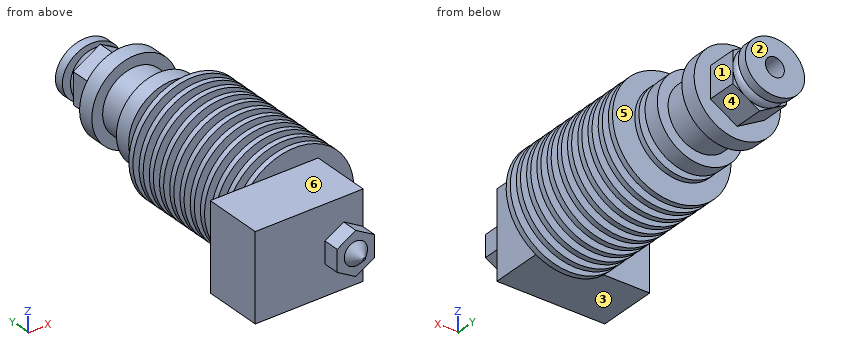
from build123d import *

# Parameters (mm, degrees)
SALIENTE_EXTRUIR1_DEPTH = 5.5
CROQUIS3_R              = 5
SALIENTE_EXTRUIR2_DEPTH = 2
REDONDEO1_R             = 2
CROQUIS4_RX             = 5.5
CROQUIS4_RY             = 5
SALIENTE_EXTRUIR3_DEPTH = 1.7
CROQUIS5_W              = 20
CROQUIS5_H              = 16
SALIENTE_EXTRUIR4_DEPTH = 11
SALIENTE_EXTRUIR5_START = 0.5
CROQUIS6_R              = 2.5
SALIENTE_EXTRUIR5_DEPTH = 0.5
SALIENTE_EXTRUIR6_DEPTH = 3
CROQUIS8_R              = 2.15
SALIENTE_EXTRUIR7_DEPTH = 2
SALIENTE_EXTRUIR7_TAPER = 44
CROQUIS9_R              = 1.75
CORTAR_EXTRUIR1_DEPTH   = 60


with BuildPart() as part:
    # Croquis1 → Revolución1 (revolve)
    with BuildSketch(Plane.XY, mode=Mode.PRIVATE) as revoluci_n1_sk:
        Polygon((0, 0), (0, 42), (8, 42), (8, 39), (6, 39), (6, 33), (8, 33), (8, 30), (4.5, 30), (4.5, 28.5), (8, 28.5), (8, 27.5), (4.5, 27.5), (4.5, 26), (11, 26), (11, 25), (4.5, 25), (4.5, 23.5), (11, 23.5), (11, 22.5), (4.5, 22.5), (4.541860465, 21), (11, 21), (11, 20), (4.569767442, 20), (4.611627907, 18.5), (11, 18.5), (11, 17.5), (4.639534884, 17.5), (4.681395349, 16), (11, 16), (11, 15), (4.709302326, 15), (4.751162791, 13.5), (11, 13.5), (11, 12.5), (4.779069767, 12.5), (4.820930233, 11), (11, 11), (11, 10), (4.848837209, 10), (4.890697674, 8.5), (11, 8.5), (11, 7.5), (4.918604651, 7.5), (4.960465116, 6), (11, 6), (11, 5), (4.988372093, 5), (5.030232558, 3.5), (11, 3.5), (11, 2.5), (5.058139535, 2.5), (5.1, 1), (11, 1), (11, 0), (2.5, 0), (2.5, -0.5), (0, -0.5), align=None)
    revolve(revoluci_n1_sk.sketch.rotate(Axis((0, 0, 0), (0, 1, 0)), 90), axis=Axis((0, 0, 0), (0, 1, 0)))

    # Croquis2 → Saliente-Extruir1 (add)
    with BuildSketch(Plane(origin=(0, 42, 0), x_dir=(1, 0, 0), z_dir=(0, 1, 0))):
        Polygon((0, 5.773502692), (-5, 2.886751346), (-5, -2.886751346), (0, -5.773502692), (5, -2.886751346), (5, 2.886751346), align=None)
    extrude(amount=SALIENTE_EXTRUIR1_DEPTH)

    # Croquis3 → Saliente-Extruir2 (add)
    with BuildSketch(Plane(origin=(0, 47.5, 0), x_dir=(1, 0, 0), z_dir=(0, 1, 0))):
        with Locations(Location((0, 0, 0), (0, 0, 60))):
            Circle(CROQUIS3_R)
    extrude(amount=SALIENTE_EXTRUIR2_DEPTH)

    # Redondeo1
    redondeo1_edges = [part.edges().sort_by_distance(p)[0] for p in [
        (-2.5, 49.5, 4.330127019),
    ]]
    fillet(redondeo1_edges, radius=REDONDEO1_R - 0.0001)  # a hair under: the kernel refuses the full size

    # Croquis4 → Saliente-Extruir3 (add)
    with BuildSketch(Plane(origin=(0, 49.5, 0), x_dir=(1, 0, 0), z_dir=(0, 1, 0))):
        with Locations(Location((0, 0), (0, 0, -180))):
            Ellipse(CROQUIS4_RX, CROQUIS4_RY)
    extrude(amount=SALIENTE_EXTRUIR3_DEPTH)

    # Croquis5 → Saliente-Extruir4 (add)
    with BuildSketch(Plane(origin=(0, -0.5, 0), x_dir=(-1, 0, 0), z_dir=(0, -1, 0))):
        with Locations((6, 0)):
            Rectangle(CROQUIS5_W, CROQUIS5_H)
    extrude(amount=SALIENTE_EXTRUIR4_DEPTH)

    # Croquis6 → Saliente-Extruir5 (add)
    with BuildSketch(Plane.XZ.offset(11.5).offset(SALIENTE_EXTRUIR5_START)):
        with Locations(Location((0, 0, 0), (0, 0, 270))):
            Circle(CROQUIS6_R)
    extrude(amount=-SALIENTE_EXTRUIR5_DEPTH)

    # Croquis7 → Saliente-Extruir6 (add)
    with BuildSketch(Plane.XZ.offset(12)):
        Polygon((0, -4), (3.464101615, -2), (3.464101615, 2), (0, 4), (-3.464101615, 2), (-3.464101615, -2), align=None)
    extrude(amount=SALIENTE_EXTRUIR6_DEPTH)

    # Croquis8 → Saliente-Extruir7 (add)
    with BuildSketch(Plane.XZ.offset(15)):
        Circle(CROQUIS8_R)
    extrude(amount=SALIENTE_EXTRUIR7_DEPTH, taper=SALIENTE_EXTRUIR7_TAPER)

    # Croquis9 → Cortar-Extruir1 (cut)
    with BuildSketch(Plane(origin=(0, 51.2, 0), x_dir=(1, 0, 0), z_dir=(0, 1, 0))):
        with Locations(Location((0, 0, 0), (0, 0, 270))):
            Circle(CROQUIS9_R)
    extrude(amount=-CORTAR_EXTRUIR1_DEPTH, mode=Mode.SUBTRACT)


solid = part.part
CAD build for the part. Positions are in the model's coordinates, mm. Face numbers are marked on the shaded views. A direction names the side the tool comes from. Coordinates: 2 decimals unless noted, no trailing zeros. Write each loop counter-clockwise with the first axis right and the second up, starting at its lowest first coordinate (ties: lowest second). Pieces come first, ordered by that corner, then holes. Notation, with made-up numbers: M 6,-17 L 54,-17 A22 cw 54,-8 Z; hole C 33.5,-21 d4. An arc over 180 degrees is marked long. Return JSON: item names as keys, results as strings.
Item 1: Which spindle directions (+Z, -Z, +X, -X, +Y, -Y) get a long thin tool onto all of the face, cutting with end or side? Do the marked faces 4, 5 and 6. Say none if no direction does.
Findings below:
{"face 4": "-Z, +X", "face 5": "none", "face 6": "+Z, +X, -X, -Y"}
Item 2: Slice it at B-B, the plane x = -14. Write the cut outline in (y, z), and give its area (3 significant figures).
Findings below:
{"outline": "M -11.5,-8 L -0.5,-8 L -0.5,8 L -11.5,8 Z", "area": "176 mm2"}
Item 3: Slice it at C-C, the plane z = -9.5. State how many separate pieces and enclosed holes the cut face has, and give its area (3 significant figures).
Findings below:
{"separate pieces": "11", "enclosed holes": "0", "area": "122 mm2"}
Item 4: Drop flat-ended pins along their axis: pin 1 Ø9 at (y, z) = (-6.5, -2) entering from +X; pin 2 Ø1.5 at (x, y) = (-5, 33) entering from -Z; pin 3 Ø5.5 at (x, y) = (-10, -8.5) entering from +Z. Give the stop position or say it passes through.
Findings below:
{"pin 1": "stops at x = 4", "pin 2": "stops at z = -6.78", "pin 3": "stops at z = 8"}
Item 5: Two-plate mould, pull along Y, no slides. Class the marked faces 1, 2 and 3: +Y half, -Y half, draft (parallel to the pull), parting line (faces both ways), or undercut.
Findings below:
{"face 1": "undercut", "face 2": "+Y half", "face 3": "draft"}
Item 6: Slice it at A-A, the plane y = 34.5. Write the cut outline in (x, z), and give its area (3 significant figures).
Findings below:
{"outline": "C 0,0 d12; hole C 0,0 d3.5", "area": "103 mm2"}
Item 7: Probe line 1 (Y direction, x = 2.5, z = -0.75); line 2 (X direction, y = 9, z = 0); line 3 (X direction, y = 18, z = 0). List the from-to ranges inside material, lowest first. Write a range as from..to.
Findings below:
{"line 1": "y = -15..-12, -11.5..-0.5, 0..51.2", "line 2": "x = -4.88..-1.75, 1.75..4.88", "line 3": "x = -11..-1.75, 1.75..11"}
